Could you check a few things on this drawing? It's one solid part, dimensions in mm from its lowest x, y, z. Give positions to 0.01 mm unless a question says otherwise; leave off trailing zeros. Order: outer loops, then holes, each group sorted by start corner. A loop starts at its lowest first (then second) coordinate and runs counter-clockwise, first axis right, second up.
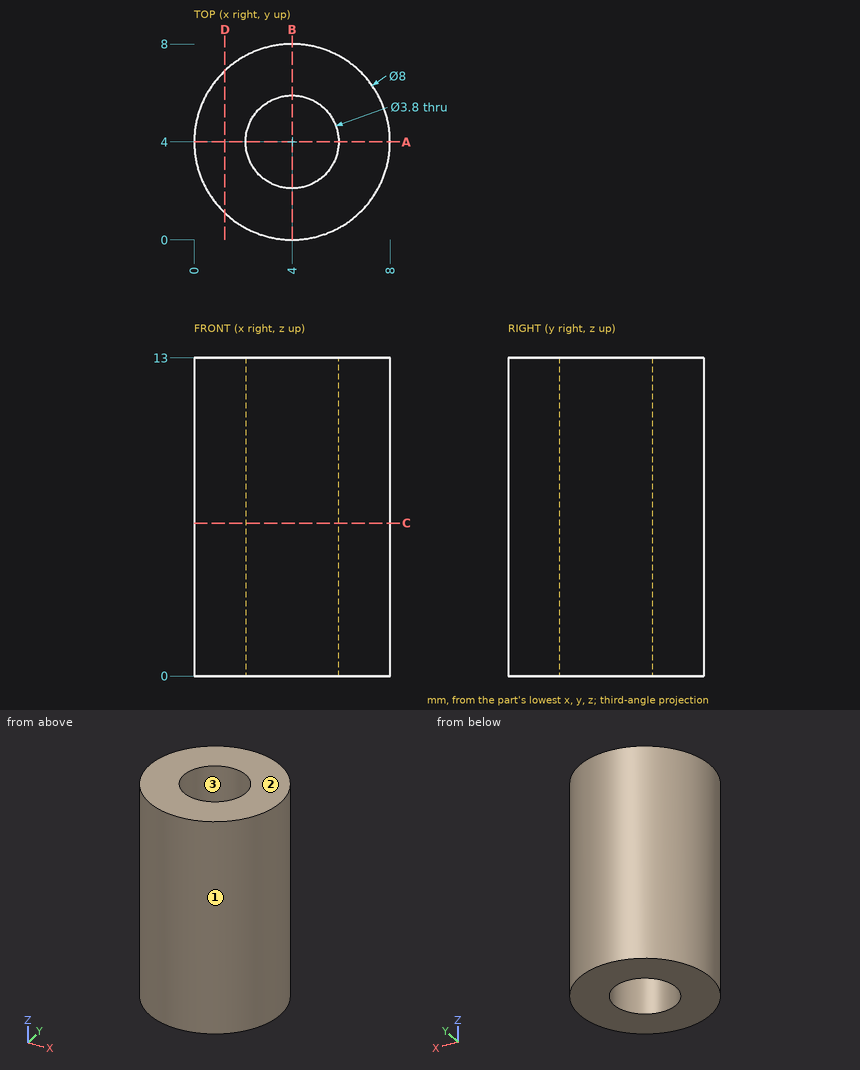
1) I'm going to push flat-ended pins straight in: pin 1 Ø1 at (x, z) = (7, 4) entering from +Y; pin 2 Ø1 at (y, z) = (3, 11) entering from +X; pin 3 Ø2 at (y, z) = (1, 4.5) entering from +X; pin 4 Ø3 at (x, y) = (4, 4) entering from -Z. Where does each tip first touch, or does it pass through?
2) If I drill on line 1 (Y direction, x = 4, z = 4.75); line 2 (Y direction, x = 4.75, z = 11.5); line 3 (X direction, y = 3.5, z = 4.75), over which ranges is the centre line in solid material (lowest first)?
3) We'd pull the mould along Y, two halves only. Please class the marked faces 1, 2 and 3: +Y half, -Y half, draft (parallel to the pull), parting line (faces both ways), or undercut.
4) Suppose I cut it at D-D (x = 1.25). Please give me the cut outline in (y, z), and give its area (3 significant figures).
5) Suppose I cut it at A-A (y = 4). Please give me the cut outline in (x, z).
6) Suppose I cut it at C-C (z = 6.25). Please give me the cut outline in (x, y), and give its area (3 significant figures).
Results:
1. pin 1: stops at y = 7.12
1. pin 2: stops at x = 7.97
1. pin 3: stops at x = 7.46
1. pin 4: passes through
2. line 1: y = 0 to 2.1, 5.9 to 8
2. line 2: y = 0.07 to 2.25, 5.75 to 7.93
2. line 3: x = 0.03 to 2.17, 5.83 to 7.97
3. face 1: parting line
3. face 2: draft
3. face 3: undercut
4. outline: (1.1, 0) - (6.9, 0) - (6.9, 13) - (1.1, 13) - close
4. area: 75.5 mm2
5. outline: (0, 0) - (2.1, 0) - (2.1, 13) - (0, 13) - close; (5.9, 0) - (8, 0) - (8, 13) - (5.9, 13) - close
6. outline: circle Ø8 at (4, 4); hole circle Ø3.8 at (4, 4)
6. area: 38.9 mm2
